Verification items for this drawing (mm, ordinates from the low corner). Coordinates: 2 decimals unless noted, no trailing zeros. Loops run counter-clockwise (first coordinate to the right, second up) from the corner with the lowest first, then second, coordinate; pieces in that order, holes last.
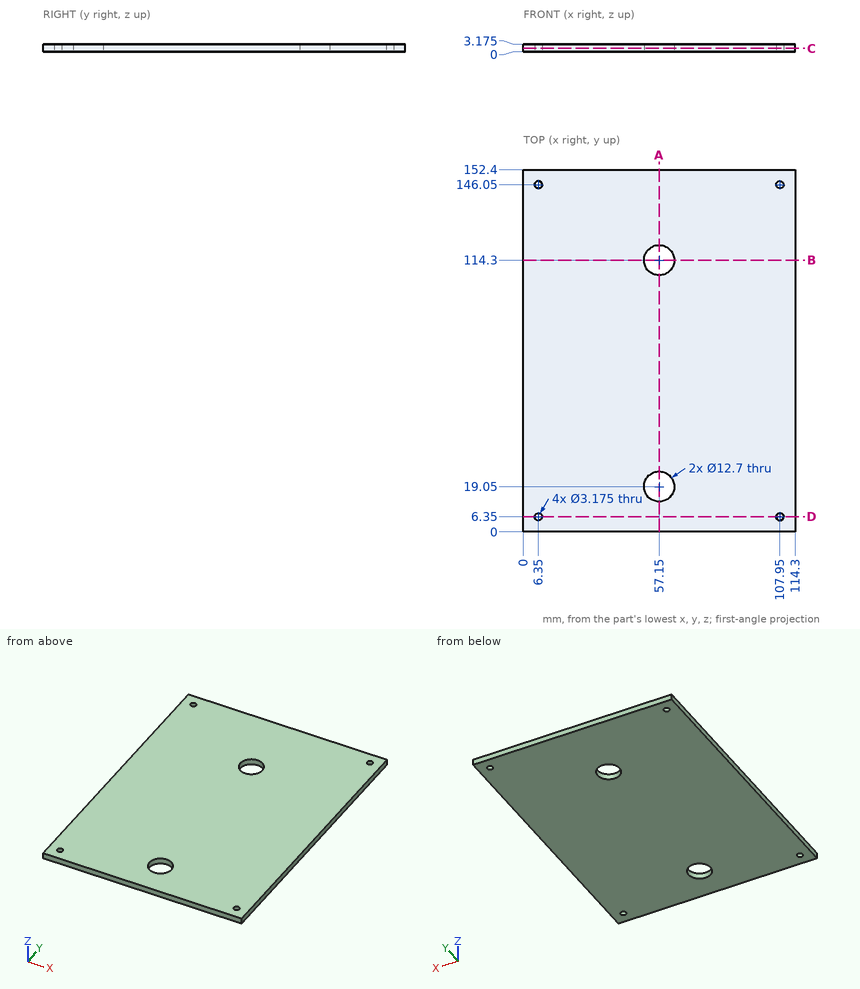
(1) Section check C-C, the plane z = 1.35. Count the separate pieces of the cut face and the enclosed holes in it, plus the area to 3 significant figures.
(2) Gauge pin test, flat ends, axial feed: P1, Ø5, axis at x = 107.95, y = 6.35, coming from the -Z side; P2, Ø7.5, axis at x = 57.15, y = 19.05, coming from the +Z side. Record the tip position at first contact, or that the pin passes through.
(3) Scan lines: line 1 along Y through (x, z) = (107.95, 1.4); line 2 along X through (y, z) = (6.35, 0.75); line 3 along Y through (x, z) = (57.15, 2.35). Record each from-to range of solid material in increasing order.
(4) Section check B-B, the plane y = 114.3. Enter the section's corners in (x, z) (3 decimals), plus the area to 3 significant figures.
(5) Section check A-A, the plane x = 57.15. Enter the section's corners in (y, z) (3 decimals).
(6) Section check D-D, the plane y = 6.35. Enter the section's corners in (x, z) (1 decimal), plus the area to 3 significant figures.
Determined:
1. separate pieces: 1
1. enclosed holes: 6
1. area: 17,100 mm2
2. P1: stops at z = 0
2. P2: passes through
3. line 1: y = 0 to 4.76, 7.94 to 144.46, 147.64 to 152.4
3. line 2: x = 0 to 4.76, 7.94 to 106.36, 109.54 to 114.3
3. line 3: y = 0 to 12.7, 25.4 to 107.95, 120.65 to 152.4
4. outline: (0, 0) - (50.8, 0) - (50.8, 3.175) - (0, 3.175) - close; (63.5, 0) - (114.3, 0) - (114.3, 3.175) - (63.5, 3.175) - close
4. area: 323 mm2
5. outline: (0, 0) - (12.7, 0) - (12.7, 3.175) - (0, 3.175) - close; (25.4, 0) - (107.95, 0) - (107.95, 3.175) - (25.4, 3.175) - close; (120.65, 0) - (152.4, 0) - (152.4, 3.175) - (120.65, 3.175) - close
6. outline: (0, 0) - (4.8, 0) - (4.8, 3.2) - (0, 3.2) - close; (7.9, 0) - (106.4, 0) - (106.4, 3.2) - (7.9, 3.2) - close; (109.5, 0) - (114.3, 0) - (114.3, 3.2) - (109.5, 3.2) - close
6. area: 343 mm2
